```python
from build123d import *

# Parameters (mm, degrees)
SKETCH1_W           = 440
SKETCH1_H           = 440
BOSS_EXTRUDE1_DEPTH = 4
SKETCH3_W           = 20
SKETCH3_H           = 20
CUT_EXTRUDE1_DEPTH  = 10
SKETCH4_R           = 6
SKETCH4_R_2         = 5
CUT_EXTRUDE2_DEPTH  = 10
SKETCH5_W           = 15
SKETCH5_H           = 400
CUT_EXTRUDE3_DEPTH  = 312.152695634


with BuildPart() as part:
    # Sketch1 → Boss-Extrude1 (new body)
    with BuildSketch(Plane(origin=(0, 0, 0), x_dir=(1, 0, 0), z_dir=(0, 1, 0))):
        Rectangle(SKETCH1_W, SKETCH1_H)
    extrude(amount=BOSS_EXTRUDE1_DEPTH)

    # Sketch3 → Cut-Extrude1 (cut)
    with BuildSketch(Plane(origin=(0, 4, 0), x_dir=(1, 0, 0), z_dir=(0, 1, 0))):
        with Locations((-210, -210)):
            Rectangle(SKETCH3_W, SKETCH3_H)
        with Locations((210, -210)):
            Rectangle(SKETCH3_W, SKETCH3_H)
        with Locations((210, 210)):
            Rectangle(SKETCH3_W, SKETCH3_H)
        with Locations((-210, 210)):
            Rectangle(SKETCH3_W, SKETCH3_H)
    extrude(amount=-CUT_EXTRUDE1_DEPTH, mode=Mode.SUBTRACT)

    # Sketch4 → Cut-Extrude2 (cut)
    with BuildSketch(Plane(origin=(0, 4, 0), x_dir=(1, 0, 0), z_dir=(0, 1, 0))):
        with Locations(Location((-147.5, 192, 0), (0, 0, 270))):
            Circle(SKETCH4_R)
        with Locations(Location((112.5, 192, 0), (0, 0, 270))):
            Circle(SKETCH4_R)
        with Locations(Location((-17.5, 185, 0), (0, 0, 270))):
            Circle(SKETCH4_R_2)
        with Locations(Location((112.5, -192, 0), (0, 0, 270))):
            Circle(SKETCH4_R)
        with Locations(Location((-17.5, -185, 0), (0, 0, 270))):
            Circle(SKETCH4_R_2)
        with Locations(Location((-147.5, -192, 0), (0, 0, 270))):
            Circle(SKETCH4_R)
    extrude(amount=-CUT_EXTRUDE2_DEPTH, mode=Mode.SUBTRACT)

    # Sketch5 → Cut-Extrude3 (cut, through all)
    with BuildSketch(Plane(origin=(0, 4, 0), x_dir=(1, 0, 0), z_dir=(0, 1, 0))):
        with Locations((212.5, 0)):
            Rectangle(SKETCH5_W, SKETCH5_H)
    extrude(amount=-CUT_EXTRUDE3_DEPTH, mode=Mode.SUBTRACT)


solid = part.part
```
Geometry check sheet. Reference: the model listing, model coordinates, mm. Round coordinates to 2 decimals unless told otherwise and drop trailing zeros. Loops run counter-clockwise (first coordinate to the right, second up) from the corner with the lowest first, then second, coordinate; pieces in that order, holes last. Notation, with made-up numbers: (-35.75, -35) - (-2.75, -35) arc R23 ccw to (-2.75, -13) - close; hole circle Ø8 at (86, 32.5). An arc over 180 degrees is marked (long way). Write item = value, one per line. Start each with the question number.
1. Depth check by flat-ended pin: pin 1 (8 mm diameter, centred on x = -17.5, z = 185, fed in from +Y); pin 2 (2 mm diameter, centred on x = -212, y = 2.5, fed in from -Z); pin 3 (1.2 mm diameter, centred on x = -209, y = 1.5, fed in from +Z); pin 4 (2 mm diameter, centred on y = 1, z = -211.5, fed in from -X). Enter the tip coordinate at first touch or a pass-through.
2. Section check A-A on x = -17.5. Enter the section's corners in (y, z), then the cut area to 3 significant figures.
3. Thickness scan on line 1 (X direction, y = 1.7, z = -192); line 2 (Z direction, x = 112, y = 0.4); line 3 (X direction, y = 1.2, z = -194). Record the ranges inside material, lowest first.
4. Section check B-B on x = -147.5. Enter the section's corners in (y, z).
5. Mould release check, pull along Z, two halves, no side actions. Record for faces 1 (the face through (-20.5, 2, 181)), 2 (the face through (-10, 4, -3)), 3 (the face through (-151.15, 2.03, -196.76)): released by +Z, released by -Z, zero draft, split by the parting line, or undercut.
Working result:
q1.pin_1 = through
q1.pin_2 = -200
q1.pin_3 = 200
q1.pin_4 = -200
q2.outline = (0, -220) - (4, -220) - (4, -190) - (0, -190) - close; (0, -180) - (4, -180) - (4, 180) - (0, 180) - close; (0, 190) - (4, 190) - (4, 220) - (0, 220) - close
q2.area = 1,680 mm^2
q3.line_1 = -220 to -153.5, -141.5 to 106.5, 118.5 to 205
q3.line_2 = -220 to -197.98, -186.02 to 186.02, 197.98 to 220
q3.line_3 = -220 to -153.16, -141.84 to 106.84, 118.16 to 205
q4.outline = (0, -220) - (4, -220) - (4, -198) - (0, -198) - close; (0, -186) - (4, -186) - (4, 186) - (0, 186) - close; (0, 198) - (4, 198) - (4, 220) - (0, 220) - close
q5.face_1 = undercut
q5.face_2 = zero draft
q5.face_3 = undercut
